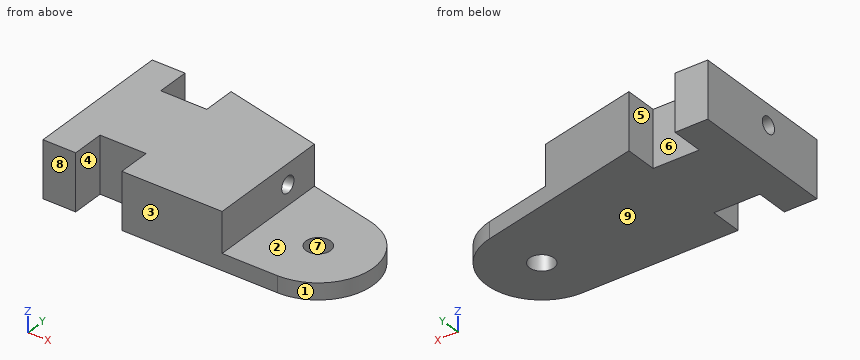
from build123d import *

# Parameters (mm, degrees)
SKETCH1_R               = 1.5
BOSS_EXTRUDE1_DEPTH     = 6.9
CUT_EXTRUDE2_DEPTH      = 4.9
SKETCH5_R               = 1
CUT_EXTRUDE3_DEPTH      = 7
SKETCH7_R               = 1
CUT_EXTRUDE4_DEPTH      = 1
CUT_EXTRUDE4_DEPTH_BACK = 29.832817126


with BuildPart() as part:
    # Sketch1 → Boss-Extrude1 (new body)
    with BuildSketch(Plane.XY):
        with BuildLine():
            Line((0, 0), (0, 18.000341084))
            Line((0, 18.000341084), (4, 18.000341084))
            Line((4, 18.000341084), (4, 14.000341084))
            Line((4, 14.000341084), (9.631516349, 14.000341084))
            Line((9.631516349, 14.000341084), (9.631516349, 18.000341084))
            Line((9.631516349, 18.000341084), (30.123176491, 13.320805491))
            ThreePointArc((30.123176491, 13.320805491), (35.324106187, 5.989458303), (28.621516349, 0))
            Line((28.621516349, 0), (9.631516349, 0))
            Line((9.631516349, 0), (9.631516349, 4))
            Line((9.631516349, 4), (4, 4))
            Line((4, 4), (4, 0))
            Line((4, 0), (0, 0))
        make_face()
        with Locations((28.621516349, 6.745044143)):
            Circle(SKETCH1_R, mode=Mode.SUBTRACT)
    extrude(amount=BOSS_EXTRUDE1_DEPTH)

    # Sketch4 → Cut-Extrude2 (cut)
    with BuildSketch(Plane.XY.offset(6.9)):
        with BuildLine():
            Line((21.876472206, 0), (21.876472206, 15.204047061))
            Line((21.876472206, 15.204047061), (30.123176491, 13.320805491))
            ThreePointArc((30.123176491, 13.320805491), (35.324106187, 5.989458303), (28.621516349, 0))
            Line((28.621516349, 0), (21.876472206, 0))
        make_face()
    extrude(amount=-CUT_EXTRUDE2_DEPTH, mode=Mode.SUBTRACT)

    # Sketch5 → Cut-Extrude3 (cut)
    with BuildSketch(Plane.ZY):
        with Locations((4.45, 8)):
            Circle(SKETCH5_R)
    extrude(amount=-CUT_EXTRUDE3_DEPTH, mode=Mode.SUBTRACT)

    # Sketch7 → Cut-Extrude4 (cut, two sides)
    with BuildSketch(Plane(origin=(8.983585976, 1.584048591, 0), x_dir=(0, 0, 1), z_dir=(-0.984807753, -0.173648178, 0))) as cut_extrude4_sk:
        with Locations((4.45, 6.87)):
            Circle(SKETCH7_R)
    extrude(amount=CUT_EXTRUDE4_DEPTH, mode=Mode.SUBTRACT)
    extrude(cut_extrude4_sk.sketch, amount=-CUT_EXTRUDE4_DEPTH_BACK, mode=Mode.SUBTRACT)


solid = part.part
For this review, take the finished solid that the model builds, in its own axes (mm). Face numbers are marked on the shaded views. A direction names the side the tool comes from. Round coordinates to 2 decimals unless told otherwise and drop trailing zeros. Write each loop counter-clockwise with the first axis right and the second up, starting at its lowest first coordinate (ties: lowest second). Pieces come first, ordered by that corner, then holes. Notation, with made-up numbers: (0, 68.5) -> (44, 68.5) arc R19 cw to (44, 76.5) -> close; hole circle Ø11 at (21.5, 71.5). An arc over 180 degrees is marked (long way). Put each result on its own line as item: value.
Q1. The part is to be moulded in two halves that separate along Y. For the marked faces 6, 7, 8 and 9, say which applies: released by +Y, released by -Y, zero draft, split by the parting line, or undercut.
Determined:
face 6: released by +Y
face 7: undercut
face 8: released by -Y
face 9: zero draft
Q2. Clearance check with flat-ended pins moving along their axes: pin 1 Ø3 at (y, z) = (5, 2) entering from +X; pin 2 Ø4 at (y, z) = (10.5, 3.5) entering from +X; pin 3 Ø1 at (x, z) = (21.5, 2.5) entering from +Y. State where each tip first meets the part, or that it passes through.
Determined:
pin 1: stops at x = 35.36
pin 2: stops at x = 34.91
pin 3: stops at y = 15.4
Q3. Consider section A-A on y = 1.5. State the section outline as (x, z) points, and give its area (3 significant figures).
Determined:
outline: (0, 0) -> (4, 0) -> (4, 6.9) -> (0, 6.9) -> close; (9.63, 0) -> (32.86, 0) -> (32.86, 2) -> (21.88, 2) -> (21.88, 6.9) -> (9.63, 6.9) -> close
area: 134 mm^2
Q4. Machinability: for the marked faces 1, 2, 3, 4 and 5, which of the approach directions +Z, -Z, +X, -X, +Y, -Y give a long, thin tool a straight path to every point of the face, cutting with its end or side? Answer none if there is none.
Determined:
face 1: +Z, -Z, +X
face 2: +Z, +X, +Y, -Y
face 3: +Z, -Z, +X, -X, -Y
face 4: +Z, -Z, -Y
face 5: +Z, -Z, +Y
Q5. Consider section B-B on z = 3. State the section outline as (x, y) points.
Determined:
outline: (0, 0) -> (4, 0) -> (4, 4) -> (9.63, 4) -> (9.63, 0) -> (21.88, 0) -> (21.88, 15.2) -> (9.63, 18) -> (9.63, 14) -> (4, 14) -> (4, 18) -> (0, 18) -> close
Q6. Consider section C-C on z = 4.45. State the section outline as (x, y) points.
Determined:
outline: (0, 0) -> (4, 0) -> (4, 4) -> (9.63, 4) -> (9.63, 0) -> (21.88, 0) -> (21.88, 9.82) -> (7, 7.19) -> (7, 7) -> (0, 7) -> close; (0, 9) -> (6.66, 9) -> (6.63, 9.16) -> (21.88, 11.85) -> (21.88, 15.2) -> (9.63, 18) -> (9.63, 14) -> (4, 14) -> (4, 18) -> (0, 18) -> close
Q7. To check wall thickness, follow L1, parallel to Z at x = 3, y = 8; L2, parallel to X at y = 2.25, z = 3.25; L3, parallel to Z at x = 23.5, y = 2.5. State the ranges of each line that lie inside material, in increasing order. Write a range as [from, to].
Determined:
L1: z = [0, 3.45], [5.45, 6.9]
L2: x = [0, 4], [9.63, 21.88]
L3: z = [0, 2]
Q8. Consider section D-D on x = 4.5. State the section outline as (y, z) points.
Determined:
outline: (4, 0) -> (14, 0) -> (14, 6.9) -> (4, 6.9) -> close; hole circle Ø2 at (8, 4.45)
